Design review of the part built by this model. Coordinates are the model's own, in mm. A direction names the side the tool comes from. Coordinates: 2 decimals unless noted, no trailing zeros. Order: outer loops, then holes, each group sorted by start corner. A loop starts at its lowest first (then second) coordinate and runs counter-clockwise, first axis right, second up. Notation, with made-up numbers: (-17, -38) - (17, -38) arc R9 ccw to (17, -21) - close; hole circle Ø10 at (56.25, -3.5). An arc over 180 degrees is marked (long way). Write each question's results on one line, items separated by ' | '. Start each with the question number.
```python
from build123d import *

# Parameters (mm, degrees)
F0_R     = 1.5
F1_DEPTH = 25
F0_R_2   = 2.94
F2_DEPTH = 12.5
F0_R_3   = 6
F3_DEPTH = 5.37
F4_R     = 0.75


with BuildPart() as f1:
    # F0 (on Top) → F1 (new body)
    with BuildSketch(Plane.XY):
        Circle(F0_R)
    extrude(amount=F1_DEPTH)

    # F0 (on Top) → F2 (join)
    with BuildSketch(Plane.XY):
        Circle(F0_R_2)
        Circle(F0_R, mode=Mode.SUBTRACT)
    extrude(amount=F2_DEPTH)

    # F0 (on Top) → F3 (join)
    with BuildSketch(Plane.XY):
        Circle(F0_R_3)
        Circle(F0_R_2, mode=Mode.SUBTRACT)
    extrude(amount=F3_DEPTH)

    # F4
    f4_edges = [f1.edges().sort_by_distance(p)[0] for p in [
        (-6, 0, 5.37),
    ]]
    fillet(f4_edges, radius=F4_R)


solid = f1.part
```
(1) Take a section at D-D (z = 1.75). State the section outline as (x, y) points, plus the area to 3 significant figures.
(2) Take a section at A-A (x = 0). State the section outline as (y, z) points.
(3) Tool access review of faces 1 (the face through (1.3, -1.3, 12.5)), 2 (the face through (0, 0, 25)): name each direction out of +Z, -Z, +X, -X, +Y, -Y from which nothing blocks a thin tool from reaching the whole face with its end or side.
(4) To check wall thickness, follow line 1 along Z through (x, y) = (-3, -3.25); line 2 along Z through (x, y) = (1, -2.5); line 3 along Y through (x, z) = (-1.25, 2.5). State the ranges of each line that lie inside material, in increasing order. Write a range as [from, to].
(5) Clearance check with flat-ended pins moving along their axes: pin 1 (1 mm diameter, centred on y = -3, z = 22.5, fed in from +X); pin 2 (1.5 mm diameter, centred on x = -2.5, z = 7, fed in from -Y); pin 3 (6 mm diameter, centred on x = 4, z = 17.5, fed in from +Y). State where each tip first meets the part, or that it passes through.
(6) Take a section at C-C (z = 13.75). State the section outline as (x, y) points, plus the area to 3 significant figures.
Worked out:
1) outline: circle Ø12 at (0, 0) | area: 113 mm^2
2) outline: (-6, 0) - (6, 0) - (6, 4.62) arc R0.75 ccw to (5.25, 5.37) - (2.94, 5.37) - (2.94, 12.5) - (1.5, 12.5) - (1.5, 25) - (-1.5, 25) - (-1.5, 12.5) - (-2.94, 12.5) - (-2.94, 5.37) - (-5.25, 5.37) arc R0.75 ccw to (-6, 4.62) - close
3) face 1: +Z | face 2: +Z, +X, -X, +Y, -Y
4) line 1: [0, 5.37] | line 2: [0, 12.5] | line 3: [-5.87, 5.87]
5) pin 1: through | pin 2: y = -2.36 | pin 3: y = 1.12
6) outline: circle Ø3 at (0, 0) | area: 7.07 mm^2
